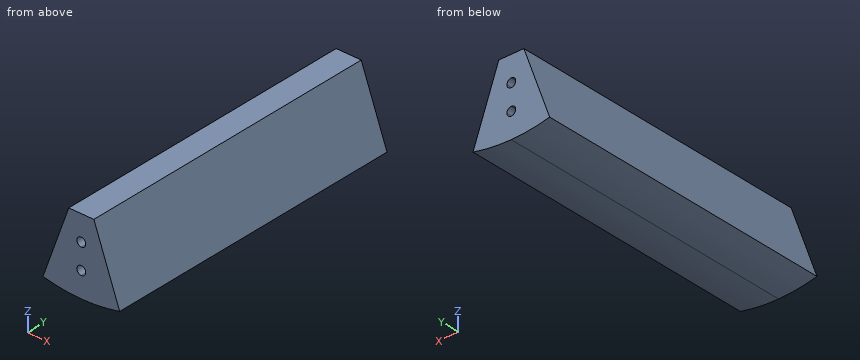
from build123d import *

# Parameters (mm, degrees)
BOSS_EXTRUDE1_DEPTH = 121.65


with BuildPart() as part:
    # Sketch1 → Boss-Extrude1 (new body)
    with BuildSketch(Plane(origin=(0, 0, 0), x_dir=(1, 0, 0), z_dir=(0, 1, 0))):
        with BuildLine():
            Line((-5, 36.5), (0, 36.5))
            Line((0, 36.5), (0, 44.75))
            ThreePointArc((0, 44.75), (-1.75, 46.5), (0, 48.25))
            Line((0, 48.25), (0, 54.75))
            ThreePointArc((0, 54.75), (-1.75, 56.5), (0, 58.25))
            Line((0, 58.25), (0, 66.5))
            ThreePointArc((0, 66.5), (-7.687629304, 66.05414715), (-15.272174355, 64.722567088))
            Line((-15.272174355, 64.722567088), (-5, 36.5))
        make_face()
        with BuildLine():
            Line((0, 44.75), (0, 36.5))
            Line((0, 36.5), (5, 36.5))
            Line((5, 36.5), (15.272174355, 64.722567088))
            ThreePointArc((15.272174355, 64.722567088), (7.687629304, 66.05414715), (0, 66.5))
            Line((0, 66.5), (0, 58.25))
            ThreePointArc((0, 58.25), (1.237436867, 57.737436867), (1.75, 56.5))
            ThreePointArc((1.75, 56.5), (1.237436867, 55.262563133), (0, 54.75))
            Line((0, 54.75), (0, 48.25))
            ThreePointArc((0, 48.25), (1.237436867, 47.737436867), (1.75, 46.5))
            ThreePointArc((1.75, 46.5), (1.237436867, 45.262563133), (0, 44.75))
        make_face()
    extrude(amount=BOSS_EXTRUDE1_DEPTH)


solid = part.part
Verification items for the finished model (mm, model axes). Give positions to 0.01 mm unless a question says otherwise; leave off trailing zeros. Loops run counter-clockwise (first coordinate to the right, second up) from the corner with the lowest first, then second, coordinate; pieces in that order, holes last.
1. Cross-section at C-C on x = 7. Record the cut outline in (y, z).
Derived:
outline: (0, -66.13) - (121.65, -66.13) - (121.65, -41.99) - (0, -41.99) - close
2. Cross-section at A-A on y = 64. Record the cut outline in (x, z).
Derived:
outline: (-15.27, -64.72) arc R66.5 ccw to (15.27, -64.72) - (5, -36.5) - (-5, -36.5) - close; hole circle Ø3.5 at (0, -56.5); hole circle Ø3.5 at (0, -46.5)
3. Go/stop test with flat-tipped pins: P1, Ø8, axis at x = -8, y = 96, coming from the -Z side; P2, Ø4, axis at y = 76, z = -44.5, coming from the +X side; P3, Ø3, axis at x = -6.5, y = 64.5, coming from the -Z side; P4, Ø1.5, axis at x = 2.5, z = -56, coming from the -Y side. Record where each tip stops, or that it passes through.
Derived:
P1: stops at z = -66.38
P2: stops at x = 8.64
P3: stops at z = -66.31
P4: stops at y = 0
4. Cross-section at B-B on z = -59.5. Record the cut outline in (x, y), and give its area (3 significant figures).
Derived:
outline: (-13.37, 0) - (13.37, 0) - (13.37, 121.65) - (-13.37, 121.65) - close
area: 3,250 mm2
5. Material ranges on probe 1 along X at (y, z) = (106.5, -57); probe 2 along Z at (x, y) = (-1, 77); probe 3 along X at (y, z) = (76, -57.5), recorded low to high.
Derived:
probe 1: x = -12.46 to -1.68, 1.68 to 12.46
probe 2: z = -66.49 to -57.94, -55.06 to -47.94, -45.06 to -36.5
probe 3: x = -12.64 to -1.44, 1.44 to 12.64
